Here's how the part is built. I have some questions about the finished solid (model axes, mm). Give positions to 0.01 mm unless a question says otherwise; leave off trailing zeros. Write each loop counter-clockwise with the first axis right and the second up, starting at its lowest first coordinate (ties: lowest second). Pieces come first, ordered by that corner, then holes. Notation, with made-up numbers: (-30, 19.5) -> (-8, 19.5) arc R22 ccw to (-8, 49.5) -> close; hole circle Ø8 at (8, 82.5). An arc over 180 degrees is marked (long way). Use one line per item in the form item = value.
```python
from build123d import *

# Parameters (mm, degrees)
SKETCH1_R           = 69.85
SKETCH1_R_2         = 63.5
BOSS_EXTRUDE1_DEPTH = 6.35
SKETCH2_R           = 2.085
CUT_EXTRUDE1_DEPTH  = 21.336


with BuildPart() as part:
    # Sketch1 → Boss-Extrude1 (new body)
    with BuildSketch(Plane.XY):
        with Locations((26.627424347, 39.834794984)):
            Circle(SKETCH1_R)
        with Locations((26.627424347, 39.834794984)):
            Circle(SKETCH1_R_2, mode=Mode.SUBTRACT)
    extrude(amount=BOSS_EXTRUDE1_DEPTH)

    # Sketch2 → Cut-Extrude1 (cut)
    with BuildSketch(Plane.XY.offset(6.35)):
        with Locations((26.627424347, 106.509794984)):
            Circle(SKETCH2_R)
        with Locations((84.369668144, 73.172294984)):
            Circle(SKETCH2_R)
        with Locations((84.369668144, 6.497294984)):
            Circle(SKETCH2_R)
        with Locations((26.627424347, -26.840205016)):
            Circle(SKETCH2_R)
        with Locations((-31.11481945, 6.497294984)):
            Circle(SKETCH2_R)
        with Locations((-31.11481945, 73.172294984)):
            Circle(SKETCH2_R)
    extrude(amount=-CUT_EXTRUDE1_DEPTH, mode=Mode.SUBTRACT)


solid = part.part
```
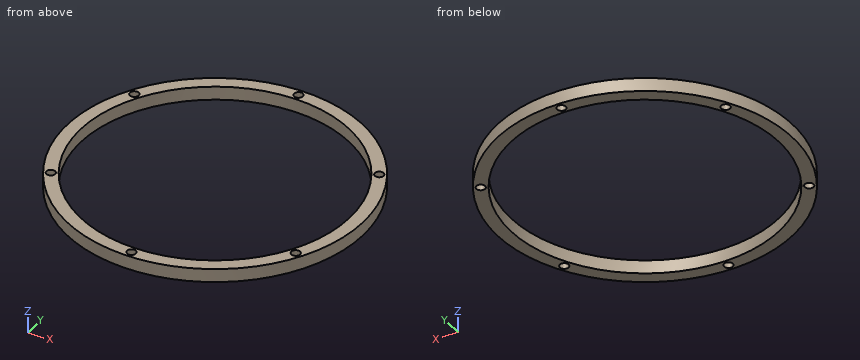
Q1. Will these pins go through, and if not, where does the flat tip stop? pin 1 Ø1 at (x, z) = (34, 3) entering from +Y; pin 2 Ø6.5 at (x, y) = (84.37, 6.5) entering from +Z; pin 3 Ø2 at (y, z) = (60.5, 3) entering from +X.
Result set:
pin_1 = 109.35
pin_2 = 6.35
pin_3 = 93.65
Q2. If I drill on line 1 along X through (y, z) = (-4.5, 4.25); line 2 along X through (y, z) = (71.5, 3.25); line 3 along Y through (x, z) = (40, 4.5), over which ranges is the centre line in solid material (lowest first)? Write a range as from..to.
Result set:
line_1 = -27.35..-18.83, 72.09..80.6
line_2 = -35.63..-32.36, -29.87..-28.41, 81.67..83.12, 85.61..88.89
line_3 = -28.72..-22.24, 101.91..108.39
Q3. I want a section at B-B, the plane x = 59. Write out the boundary of the cut face in (y, z), and give its area (3 significant figures).
Result set:
outline = (-22.06, 0) -> (-14.79, 0) -> (-14.79, 6.35) -> (-22.06, 6.35) -> close; (94.46, 0) -> (101.73, 0) -> (101.73, 6.35) -> (94.46, 6.35) -> close
area = 92.3 mm2
Q4. I want a section at A-A, the plane y = 88. Write out the boundary of the cut face in (x, z).
Result set:
outline = (-23.96, 0) -> (-14.75, 0) -> (-14.75, 6.35) -> (-23.96, 6.35) -> close; (68.01, 0) -> (77.22, 0) -> (77.22, 6.35) -> (68.01, 6.35) -> close
Q5. I want a section at C-C, the plane z = 4. Write out the boundary of the cut face in (x, y) (3 decimals), and give its area (3 significant figures).
Result set:
outline = circle Ø139.7 at (26.627, 39.835); hole circle Ø127 at (26.627, 39.835); hole circle Ø4.17 at (-31.115, 6.497); hole circle Ø4.17 at (-31.115, 73.172); hole circle Ø4.17 at (26.627, -26.84); hole circle Ø4.17 at (26.627, 106.51); hole circle Ø4.17 at (84.37, 6.497); hole circle Ø4.17 at (84.37, 73.172)
area = 2,580 mm2
Q6. I want a section at D-D, the plane x = 84. Write out the boundary of the cut face in (y, z).
Result set:
outline = (-0.01, 0) -> (4.45, 0) -> (4.45, 6.35) -> (-0.01, 6.35) -> close; (8.55, 0) -> (12.62, 0) -> (12.62, 6.35) -> (8.55, 6.35) -> close; (67.05, 0) -> (71.12, 0) -> (71.12, 6.35) -> (67.05, 6.35) -> close; (75.22, 0) -> (79.68, 0) -> (79.68, 6.35) -> (75.22, 6.35) -> close
